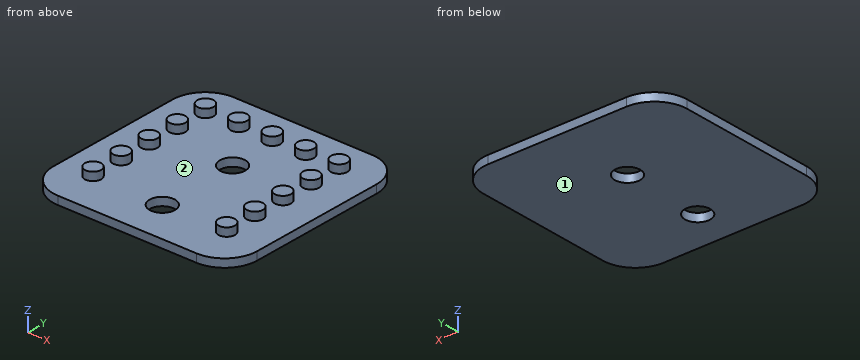
```python
from build123d import *

# Parameters (mm, degrees)
SKETCH1_W           = 25
SKETCH1_H           = 25
BOSS_EXTRUDE1_DEPTH = 1
SKETCH2_R           = 1
BOSS_EXTRUDE2_DEPTH = 1
FILLET1_R           = 4
CUT_EXTRUDE1_REACH  = 3
SKETCH3_R           = 1.55


with BuildPart() as part:
    # Sketch1 → Boss-Extrude1 (new body)
    with BuildSketch(Plane.XY):
        with Locations((-23.5, 20.5)):
            Rectangle(SKETCH1_W, SKETCH1_H)
    extrude(amount=BOSS_EXTRUDE1_DEPTH)

    # Sketch2 → Boss-Extrude2 (add)
    with BuildSketch(Plane.XY.offset(1)):
        with Locations((-32, 29)):
            Circle(SKETCH2_R)
        with Locations((-27.9, 29)):
            Circle(SKETCH2_R)
        with Locations((-23.8, 29)):
            Circle(SKETCH2_R)
        with Locations((-19.7, 29)):
            Circle(SKETCH2_R)
        with Locations((-15.6, 29)):
            Circle(SKETCH2_R)
        with Locations((-32, 25)):
            Circle(SKETCH2_R)
        with Locations((-15.6, 25)):
            Circle(SKETCH2_R)
        with Locations((-32, 21)):
            Circle(SKETCH2_R)
        with Locations((-15.6, 21)):
            Circle(SKETCH2_R)
        with Locations((-32, 17)):
            Circle(SKETCH2_R)
        with Locations((-15.6, 17)):
            Circle(SKETCH2_R)
        with Locations((-32, 13)):
            Circle(SKETCH2_R)
        with Locations((-15.6, 13)):
            Circle(SKETCH2_R)
    extrude(amount=BOSS_EXTRUDE2_DEPTH)

    # Fillet1
    fillet1_edges = [part.edges().sort_by_distance(p)[0] for p in [
        (-11, 8, 0.5),
        (-36, 8, 0.5),
        (-36, 33, 0.5),
        (-11, 33, 0.5),
    ]]
    fillet(fillet1_edges, radius=FILLET1_R)

    # Sketch3 → Cut-Extrude1 (cut, up to next)
    with BuildSketch(Plane.XY.offset(1), mode=Mode.PRIVATE) as cut_extrude1_sk1:
        with Locations((-23.5, 23)):
            Circle(SKETCH3_R)
    cut_extrude1_tool1 = extrude(cut_extrude1_sk1.sketch, amount=-CUT_EXTRUDE1_REACH, mode=Mode.PRIVATE) & part.part
    add(cut_extrude1_tool1.solids().sort_by_distance((-23.5, 23, 1))[0], mode=Mode.SUBTRACT)
    # Sketch3 → Cut-Extrude1 (cut, up to next)
    with BuildSketch(Plane.XY.offset(1), mode=Mode.PRIVATE) as cut_extrude1_sk2:
        with Locations((-23.5, 13)):
            Circle(SKETCH3_R)
    cut_extrude1_tool2 = extrude(cut_extrude1_sk2.sketch, amount=-CUT_EXTRUDE1_REACH, mode=Mode.PRIVATE) & part.part
    add(cut_extrude1_tool2.solids().sort_by_distance((-23.5, 13, 1))[0], mode=Mode.SUBTRACT)


solid = part.part
```
For this review, take the finished solid that the model builds, in its own axes (mm). Face numbers are marked on the shaded views. Round coordinates to 2 decimals unless told otherwise and drop trailing zeros. Order: outer loops, then holes, each group sorted by start corner. A loop starts at its lowest first (then second) coordinate and runs counter-clockwise, first axis right, second up. Notation, with made-up numbers: (55.5, 60.25) -> (71.5, 60.25) arc R31 ccw to (71.5, 89.25) -> close; hole circle Ø8 at (-5, -8.5). An arc over 180 degrees is marked (long way). Use a Markdown table: item, result.
Item 1: Take a section at A-A (y = 13). State the section outline as (x, z) points, plus the area to 3 significant figures.
Resolved:
| item | result |
|---|---|
| outline | (-36, 0) -> (-25.05, 0) -> (-25.05, 1) -> (-31, 1) -> (-31, 2) -> (-33, 2) -> (-33, 1) -> (-36, 1) -> close; (-21.95, 0) -> (-11, 0) -> (-11, 1) -> (-14.6, 1) -> (-14.6, 2) -> (-16.6, 2) -> (-16.6, 1) -> (-21.95, 1) -> close |
| area | 25.9 mm² |
Item 2: Take a section at D-D (y = 23). State the section outline as (x, z) points.
Resolved:
| item | result |
|---|---|
| outline | (-36, 0) -> (-25.05, 0) -> (-25.05, 1) -> (-36, 1) -> close; (-21.95, 0) -> (-11, 0) -> (-11, 1) -> (-21.95, 1) -> close |
Item 3: Draft analysis for pull direction X (two halves, no side actions). For the marked faces 1 and 2, state which applies: +X half, -X half, draft (parallel to the pull), parting line (faces both ways), or undercut.
Resolved:
| item | result |
|---|---|
| face 1 | draft |
| face 2 | undercut |
Item 4: Take a section at C-C (x = -15.6). State the section outline as (y, z) points, plus the area to 3 significant figures.
Resolved:
| item | result |
|---|---|
| outline | (8, 0) -> (33, 0) -> (33, 1) -> (30, 1) -> (30, 2) -> (28, 2) -> (28, 1) -> (26, 1) -> (26, 2) -> (24, 2) -> (24, 1) -> (22, 1) -> (22, 2) -> (20, 2) -> (20, 1) -> (18, 1) -> (18, 2) -> (16, 2) -> (16, 1) -> (14, 1) -> (14, 2) -> (12, 2) -> (12, 1) -> (8, 1) -> close |
| area | 35.0 mm² |
Item 5: Take a section at B-B (z = 1.6). State how many separate pieces and enclosed holes the cut face has, plus the area to 3 significant figures.
Resolved:
| item | result |
|---|---|
| separate pieces | 13 |
| enclosed holes | 0 |
| area | 40.8 mm² |
Item 6: For pin 1 (4 mm diameter, centred on x = -19.5, y = 13, fed in from -Z); pin 2 (8 mm diameter, centred on x = -27, y = 23, fed in from +Z), all flat-tipped, find the tip position at first contact; note any pin that passes through.
Resolved:
| item | result |
|---|---|
| pin 1 | stops at z = 0 |
| pin 2 | stops at z = 1 |
Item 7: For line 1 along Y through (x, z) = (-23.5, 0.45); line 2 along Z through (x, y) = (-28.25, 14.5); line 3 along X through (y, z) = (14, 0.65), list the stretches that pass through material, from the lowest coordinate up. Write a range as [from, to].
Resolved:
| item | result |
|---|---|
| line 1 | y = [8, 11.45], [14.55, 21.45], [24.55, 33] |
| line 2 | z = [0, 1] |
| line 3 | x = [-36, -24.68], [-22.32, -11] |
